from build123d import *

# Parameters (mm, degrees)
SKETCH1_W           = 508
SKETCH1_H           = 635
BOSS_EXTRUDE1_DEPTH = 6.35
SKETCH3_W           = 508
SKETCH3_H           = 298.45
BOSS_EXTRUDE3_DEPTH = 6.35
BOSS_EXTRUDE4_DEPTH = 12.7
SKETCH6_W           = 298.45
SKETCH6_H           = 25.4
BOSS_EXTRUDE6_DEPTH = 482.6
CUT_EXTRUDE1_DEPTH  = 25.4


with BuildPart() as part:
    # Sketch1 → Boss-Extrude1 (new body)
    with BuildSketch(Plane.XY):
        with Locations((254, 317.5)):
            Rectangle(SKETCH1_W, SKETCH1_H)
    extrude(amount=BOSS_EXTRUDE1_DEPTH)

    # Sketch3 → Boss-Extrude3 (add)
    with BuildSketch(Plane(origin=(0, 0, 0), x_dir=(1, 0, 0), z_dir=(0, 1, 0))):
        with Locations((254, -155.575)):
            Rectangle(SKETCH3_W, SKETCH3_H)
    extrude(amount=BOSS_EXTRUDE3_DEPTH)

    # Sketch4 → Boss-Extrude4 (add)
    with BuildSketch(Plane(origin=(0, 0, 0), x_dir=(0, 0, -1), z_dir=(1, 0, 0))):
        Polygon((-304.8, 6.35), (-304.8, 635), (-6.35, 635), (-6.35, 609.6), (-279.4, 609.6), (-279.4, 6.35), align=None)
    boss_extrude4 = extrude(amount=BOSS_EXTRUDE4_DEPTH)

    # Mirror1: Boss-Extrude4 across plane
    add(boss_extrude4.mirror(Plane(origin=(254, 0, 0), x_dir=(0, 0, 1), z_dir=(1, 0, 0))))

    # Sketch6 → Boss-Extrude6 (add)
    with BuildSketch(Plane(origin=(12.7, 0, 0), x_dir=(0, 0, -1), z_dir=(1, 0, 0))):
        with Locations((-155.575, 622.3)):
            Rectangle(SKETCH6_W, SKETCH6_H)
    extrude(amount=BOSS_EXTRUDE6_DEPTH)

    # Sketch7 → Cut-Extrude1 (cut)
    with BuildSketch(Plane(origin=(0, 635, 0), x_dir=(1, 0, 0), z_dir=(0, 1, 0))):
        with BuildLine():
            Line((292.1, -63.5), (292.1, -241.3))
            ThreePointArc((292.1, -241.3), (254, -279.4), (215.9, -241.3))
            Line((215.9, -241.3), (215.9, -63.5))
            ThreePointArc((215.9, -63.5), (254, -25.4), (292.1, -63.5))
        make_face()
    extrude(amount=-CUT_EXTRUDE1_DEPTH, mode=Mode.SUBTRACT)


solid = part.part
Could you check a few things on this model? Use its own coordinates, in mm. A direction names the side the tool comes from. Give positions to 0.01 mm unless a question says otherwise; leave off trailing zeros. Loops run counter-clockwise (first coordinate to the right, second up) from the corner with the lowest first, then second, coordinate; pieces in that order, holes last. Notation, with made-up numbers: M -21,53 L 1,53 A18 cw 1,73 Z; hole C 46.25,67.25 d6. An arc over 180 degrees is marked long. Answer as a JSON object with one key per item and string values.
Q1. If I drill on probe 1 along Y at (x, z) = (63, 128); probe 2 along X at (y, z) = (322.5, 282.5); probe 3 along Y at (x, z) = (244, 74.5), over which ranges is the centre line in solid material (lowest first)? Write a range as [from, to].
Values found:
{"probe 1": "y = [0, 6.35], [609.6, 635]", "probe 2": "x = [0, 12.7], [495.3, 508]", "probe 3": "y = [0, 6.35]"}
Q2. Suppose I cut it at C-C, the plane z = 200. List the corners of the cut face in (x, y) for me, plus the area to 3 significant figures.
Values found:
{"outline": "M 0,0 L 508,0 L 508,6.35 L 0,6.35 Z; M 0,609.6 L 215.9,609.6 L 215.9,635 L 0,635 Z; M 292.1,609.6 L 508,609.6 L 508,635 L 292.1,635 Z", "area": "14,200 mm²"}
Q3. For P1, Ø7.5, axis at y = 353.5, z = 295.5, coming from the -X side; P2, Ø1, axis at x = 123.5, y = 151, coming from the +Z side, each with a flat end and sliding along its axis, tell me the tip position at first contact or that it passes through.
Values found:
{"P1": "stops at x = 0", "P2": "stops at z = 6.35"}
Q4. If we mould it in two halves opening along Y, with no side actions, what happens to faces 4 (the flat face through (250, 312, 6.35)), 5 (the flat face through (250, 0, 150)), 6 (the flat face through (0, 390, 287))? For each: pulls with the +Y half, pulls with the -Y half, needs draft (parallel to the pull), parting line crosses it, or undercut.
Values found:
{"face 4": "undercut", "face 5": "pulls with the -Y half", "face 6": "needs draft"}
Q5. Suppose I cut it at B-B, the plane y = 156.5. List the corners of the cut face in (x, z) for me.
Values found:
{"outline": "M 0,0 L 508,0 L 508,6.35 L 0,6.35 Z; M 0,279.4 L 12.7,279.4 L 12.7,304.8 L 0,304.8 Z; M 495.3,279.4 L 508,279.4 L 508,304.8 L 495.3,304.8 Z"}
Q6. Suppose I cut it at A-A, the plane x = 254. List the corners of the cut face in (y, z) for me, plus the area to 3 significant figures.
Values found:
{"outline": "M 0,0 L 635,0 L 635,25.4 L 609.6,25.4 L 609.6,6.35 L 6.35,6.35 L 6.35,304.8 L 0,304.8 Z; M 609.6,279.4 L 635,279.4 L 635,304.8 L 609.6,304.8 Z", "area": "7,060 mm²"}
Q7. Suppose I cut it at D-D, the plane x = 395. List the corners of the cut face in (y, z) for me.
Values found:
{"outline": "M 0,0 L 635,0 L 635,304.8 L 609.6,304.8 L 609.6,6.35 L 6.35,6.35 L 6.35,304.8 L 0,304.8 Z"}
Q8. For faces 1 (the flat face through (253, 622, 304.8)), 2 (the flat face through (12.7, 312, 292)), 3 (the cylindrical face through (253.16, 622.48, 25.41)), which set-ups out of +Z, -Z, +X, -X, +Y, -Y let a thin tool reach every point of the face, with its end or its side?
Values found:
{"face 1": "+Z, +X, -X, +Y, -Y", "face 2": "+Z", "face 3": "+Y"}
